The model under review builds one solid part; all positions refer to its coordinate system, in mm. A direction names the side the tool comes from. Round coordinates to 2 decimals unless told otherwise and drop trailing zeros. Order: outer loops, then holes, each group sorted by start corner. A loop starts at its lowest first (then second) coordinate and runs counter-clockwise, first axis right, second up. Notation, with made-up numbers: M -0.75,16.25 L 57.25,16.25 A27 cw 57.25,43.25 Z; hole C 19.25,76.25 d8. An arc over 180 degrees is marked long. Answer as a JSON object with one key per item and string values. Group by question number.
1) Insertion check: pin 1 Ø3 at (x, z) = (-3, -44.5) entering from -Y; pin 2 Ø1.5 at (y, z) = (24, -40) entering from -X; pin 3 Ø1 at (y, z) = (7, -44.5) entering from -X; pin 4 Ø8 at (y, z) = (16.5, -41) entering from -X. Each pin has a flat end and moves straight along its axis. Give the tip position at first contact, or say it passes through.
2) For faces 1 (the cylindrical face through (5.47, 20.75, -35.1)), 2 (the flat face through (-9, 5, -38)), list the 3-axis set-ups (+Z, -Z, +X, -X, +Y, -Y) from which the entire face can be reached by the end or side of a thin tool; tool diameter is ignored.
3) Consider section D-D, the plane x = -1.75. Write out the cut boundary in (y, z), then the cut area to 3 significant figures.
4) Consider section B-B, the plane z = -36.75. Write out the cut boundary in (x, y).
5) Consider section A-A, the plane x = -13.5. Write out the cut boundary in (y, z).
6) To check wall thickness, follow line 1 (Z direction, x = 2.75, y = 12); line 2 (X direction, y = 15.5, z = -38); line 3 (Y direction, x = -14.25, z = -33.5). State the ranges of each line that lie inside material, in increasing order.
7) The part is to be moulded in two halves that separate along X. For faces 3 (the cylindrical face through (-11.25, 2.54, -35.1)), 4 (the flat face through (-4, 13, -45)), 5 (the flat face through (-1, 9, -32.485)), say which applies: +X half, -X half, draft (parallel to the pull), parting line (faces both ways), or undercut.
8) Consider section C-C, the plane y = 18. Write out the cut boundary in (x, z), then the cut area to 3 significant figures.
```python
from build123d import *

# Parameters (mm, degrees)
SKETCH2_W           = 30
SKETCH2_H           = 20
BOSS_EXTRUDE1_DEPTH = 30
SKETCH3_W           = 25
SKETCH3_H           = 10
CUT_EXTRUDE1_DEPTH  = 25
CUT_EXTRUDE3_DEPTH  = 25
CUT_EXTRUDE4_DEPTH  = 25
CUT_EXTRUDE5_DEPTH  = 25
SKETCH7_R           = 2.5
CUT_EXTRUDE6_DEPTH  = 25
SKETCH8_R           = 2.5
CUT_EXTRUDE7_DEPTH  = 25


with BuildPart() as part:
    # Sketch2 → Boss-Extrude1 (new body)
    with BuildSketch(Plane(origin=(0, 0, 0), x_dir=(1, 0, 0), z_dir=(0, 1, 0))):
        with Locations((-6.999241769, 37.48522127)):
            Rectangle(SKETCH2_W, SKETCH2_H)
    extrude(amount=BOSS_EXTRUDE1_DEPTH)

    # Sketch3 → Cut-Extrude1 (cut)
    with BuildSketch(Plane(origin=(0, 30, 0), x_dir=(1, 0, 0), z_dir=(0, 1, 0))):
        with Locations((-9.499241769, 37.48522127)):
            Rectangle(SKETCH3_W, SKETCH3_H)
    extrude(amount=-CUT_EXTRUDE1_DEPTH, mode=Mode.SUBTRACT)

    # Sketch4 → Cut-Extrude3 (cut)
    with BuildSketch(Plane(origin=(0, 0, -47.48522127), x_dir=(-1, 0, 0), z_dir=(0, 0, -1))):
        Polygon((21.999241769, 30), (-3.000758231, 30), (-3.000758231, 20), (11.999241769, 5), (21.999241769, 5), align=None)
    extrude(amount=-CUT_EXTRUDE3_DEPTH, mode=Mode.SUBTRACT)

    # Sketch5 → Cut-Extrude4 (cut)
    with BuildSketch(Plane(origin=(8.000758231, 0, 0), x_dir=(0, 0, -1), z_dir=(1, 0, 0))):
        with BuildLine():
            Line((37.48522127, 30), (27.48522127, 30))
            Line((27.48522127, 30), (27.48522127, 25))
            ThreePointArc((27.48522127, 25), (31.895051326, 28.680339887), (37.48522127, 30))
        make_face()
        with BuildLine():
            Line((47.48522127, 30), (37.48522127, 30))
            ThreePointArc((37.48522127, 30), (43.075391214, 28.680339887), (47.48522127, 25))
            Line((47.48522127, 25), (47.48522127, 30))
        make_face()
    extrude(amount=-CUT_EXTRUDE4_DEPTH, mode=Mode.SUBTRACT)

    # Sketch6 → Cut-Extrude5 (cut)
    with BuildSketch(Plane.XZ):
        with BuildLine():
            Line((-16.999241769, -27.48522127), (-21.999241769, -27.48522127))
            Line((-21.999241769, -27.48522127), (-21.999241769, -37.485221231))
            ThreePointArc((-21.999241769, -37.485221231), (-20.679581647, -31.895051309), (-16.999241769, -27.48522127))
        make_face()
        with BuildLine():
            ThreePointArc((-16.999241769, -47.48522127), (-20.679581665, -43.075391196), (-21.999241769, -37.485221231))
            Line((-21.999241769, -37.485221231), (-21.999241769, -47.48522127))
            Line((-21.999241769, -47.48522127), (-16.999241769, -47.48522127))
        make_face()
    extrude(amount=-CUT_EXTRUDE5_DEPTH, mode=Mode.SUBTRACT)

    # Sketch7 → Cut-Extrude6 (cut)
    with BuildSketch(Plane(origin=(0, 5, 0), x_dir=(1, 0, 0), z_dir=(0, 1, 0))):
        with Locations(Location((-11.999241769, 37.48522127, 0), (0, 0, 270))):
            Circle(SKETCH7_R)
    extrude(amount=-CUT_EXTRUDE6_DEPTH, mode=Mode.SUBTRACT)

    # Sketch8 → Cut-Extrude7 (cut)
    with BuildSketch(Plane.ZY.offset(-3.000758231)):
        with Locations((-37.48522127, 20)):
            Circle(SKETCH8_R)
    extrude(amount=-CUT_EXTRUDE7_DEPTH, mode=Mode.SUBTRACT)


solid = part.part
```
Results list:
{
 "1": {"pin 1": "y = 0", "pin 2": "x = 3", "pin 3": "x = -10.5", "pin 4": "x = -4.21"},
 "2": {"face 1": "+X, -X", "face 2": "-X, +Y"},
 "3": {"outline": "M 0,-47.49 L 15.25,-47.49 L 15.25,-42.49 L 5,-42.49 L 5,-32.49 L 15.25,-32.49 L 15.25,-27.49 L 0,-27.49 Z", "area": "202 mm^2"},
 "4": {"outline": "M -21.98,0 L -14.39,0 L -14.39,5 L -21.98,5 Z; M -9.61,0 L 8,0 L 8,17.61 L 3,17.61 L 3,5 L -9.61,5 Z; M 3,22.39 L 8,22.39 L 8,29.98 L 3,29.98 Z"},
 "5": {"outline": "M 0,-47.49 L 5,-47.49 L 5,-39.48 L 0,-39.48 Z; M 0,-35.49 L 5,-35.49 L 5,-27.49 L 0,-27.49 Z"},
 "6": {"line 1": "-47.49 to -42.49, -32.49 to -27.49", "line 2": "3 to 8", "line 3": "0 to 5"},
 "7": {"face 3": "undercut", "face 4": "-X half", "face 5": "draft"},
 "8": {"outline": "M 1,-47.49 L 8,-47.49 L 8,-38.99 L 3,-38.99 L 3,-42.49 L 1,-42.49 Z; M 1,-32.49 L 3,-32.49 L 3,-35.99 L 8,-35.99 L 8,-27.49 L 1,-27.49 Z", "area": "105 mm^2"}
}
